Here's how the part is built. I have some questions about the finished solid (model axes, mm). Face numbers are marked on the shaded views. Coordinates: 2 decimals unless noted, no trailing zeros. Write each question's results on one line, items separated by ' | '. Start each with the question number.
from build123d import *

# Parameters (mm, degrees)
F2_R      = 8
F3_DEPTH  = 1
F9_R      = 1
F9_R_2    = 2.6
F10_DEPTH = 5.001


with BuildPart() as f3:
    # F2 (on offset) → F3 (new body)
    with BuildSketch(Plane.XY.offset(-5)):
        Circle(F2_R)
    extrude(amount=F3_DEPTH)

    # F4 (on face) → F5 section 0
    with BuildSketch(Plane.XY.offset(-4)):
        with BuildLine():
            Line((0, 0), (5.6568542495, 5.6568542495))
            ThreePointArc((5.6568542495, 5.6568542495), (3.8674315589, 7.0030688371), (1.775, 7.8006009384))
            ThreePointArc((1.775, 7.8006009384), (0, 8), (-1.775, 7.8006009384))
            ThreePointArc((-1.775, 7.8006009384), (-3.8674315589, 7.0030688371), (-5.6568542495, 5.6568542495))
            Line((-5.6568542495, 5.6568542495), (0, 0))
        make_face()
    # F0 (on Top) → F5 section 1
    with BuildSketch(Plane.XY):
        with BuildLine():
            Line((1.775, 1.775), (1.775, 5.9926517503))
            ThreePointArc((1.775, 5.9926517503), (0, 6.25), (-1.775, 5.9926517503))
            Line((-1.775, 5.9926517503), (-1.775, 1.775))
            Line((-1.775, 1.775), (0, 0))
            Line((0, 0), (1.775, 1.775))
        make_face()
    loft()

    # F4 (on face) → F6 section 0
    with BuildSketch(Plane.XY.offset(-4)):
        with BuildLine():
            Line((-5.6568542495, -5.6568542495), (0, 0))
            Line((0, 0), (-5.6568542495, 5.6568542495))
            ThreePointArc((-5.6568542495, 5.6568542495), (-7.0030688371, 3.8674315589), (-7.8006009384, 1.775))
            ThreePointArc((-7.8006009384, 1.775), (-8, 0), (-7.8006009384, -1.775))
            ThreePointArc((-7.8006009384, -1.775), (-7.0030688371, -3.8674315589), (-5.6568542495, -5.6568542495))
        make_face()
    # F0 (on Top) → F6 section 1
    with BuildSketch(Plane.XY):
        with BuildLine():
            Line((-1.775, -1.775), (0, 0))
            Line((0, 0), (-1.775, 1.775))
            Line((-1.775, 1.775), (-5.9926517503, 1.775))
            ThreePointArc((-5.9926517503, 1.775), (-6.25, 0), (-5.9926517503, -1.775))
            Line((-5.9926517503, -1.775), (-1.775, -1.775))
        make_face()
    loft()

    # F4 (on face) → F7 section 0
    with BuildSketch(Plane.XY.offset(-4)):
        with BuildLine():
            Line((5.6568542495, -5.6568542495), (0, 0))
            Line((0, 0), (-5.6568542495, -5.6568542495))
            ThreePointArc((-5.6568542495, -5.6568542495), (-3.8674315589, -7.0030688371), (-1.775, -7.8006009384))
            ThreePointArc((-1.775, -7.8006009384), (0, -8), (1.775, -7.8006009384))
            ThreePointArc((1.775, -7.8006009384), (3.8674315589, -7.0030688371), (5.6568542495, -5.6568542495))
        make_face()
    # F0 (on Top) → F7 section 1
    with BuildSketch(Plane.XY):
        with BuildLine():
            Line((1.775, -1.775), (0, 0))
            Line((0, 0), (-1.775, -1.775))
            Line((-1.775, -1.775), (-1.775, -5.9926517503))
            ThreePointArc((-1.775, -5.9926517503), (0, -6.25), (1.775, -5.9926517503))
            Line((1.775, -5.9926517503), (1.775, -1.775))
        make_face()
    loft()

    # F4 (on face) → F8 section 0
    with BuildSketch(Plane.XY.offset(-4)):
        with BuildLine():
            ThreePointArc((7.8006009384, 1.775), (7.0030688371, 3.8674315589), (5.6568542495, 5.6568542495))
            Line((5.6568542495, 5.6568542495), (0, 0))
            Line((0, 0), (5.6568542495, -5.6568542495))
            ThreePointArc((5.6568542495, -5.6568542495), (7.0030688371, -3.8674315589), (7.8006009384, -1.775))
            ThreePointArc((7.8006009384, -1.775), (8, 0), (7.8006009384, 1.775))
        make_face()
    # F0 (on Top) → F8 section 1
    with BuildSketch(Plane.XY):
        with BuildLine():
            Line((5.9926517503, 1.775), (1.775, 1.775))
            Line((1.775, 1.775), (0, 0))
            Line((0, 0), (1.775, -1.775))
            Line((1.775, -1.775), (5.9926517503, -1.775))
            ThreePointArc((5.9926517503, -1.775), (6.25, 0), (5.9926517503, 1.775))
        make_face()
    loft()

    # F9 (on Top) → F10 (cut, through all)
    with BuildSketch(Plane.XY):
        with Locations((0, 4.5)):
            Circle(F9_R)
        with Locations((4.5, 0)):
            Circle(F9_R)
        with Locations((0, -4.5)):
            Circle(F9_R)
        with Locations((-4.5, 0)):
            Circle(F9_R)
        Circle(F9_R_2)
    extrude(amount=-F10_DEPTH, mode=Mode.SUBTRACT)


solid = f3.part
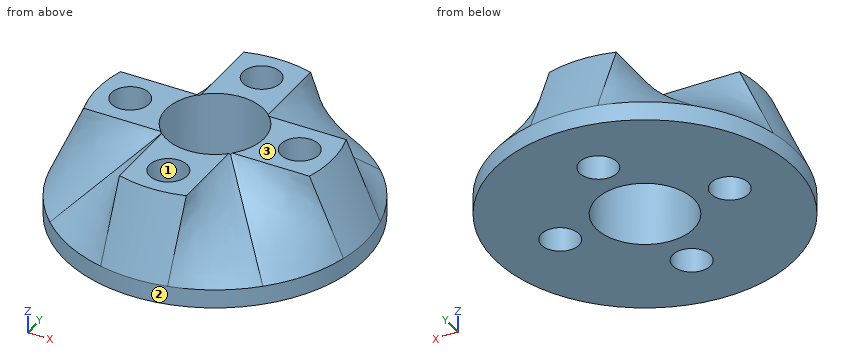
1) I want a section at A-A, the plane x = 0. Give the number of separate pieces and of enclosed holes in the cut face, then the cut area to 3 significant figures.
2) We'd pull the mould along Y, two halves only. Please class the marked faces 1, 2 and 3: pulls with the +Y half, pulls with the -Y half, needs draft (parallel to the pull), parting line crosses it, or undercut.
3) Please list where these lines run through material, in increasing order: line 1 (Y direction, x = 0, z = -1.4); line 2 (Y direction, x = 0, z = -2.4); line 3 (X direction, y = 0.25, z = -3.05). Write a range as [from, to].
4) For pin 1 Ø3 at (x, z) = (-4.5, -4) entering from +Y; pin 2 Ø1 at (x, y) = (2.5, -2.5) entering from +Z; pin 3 Ø4.5 at (x, y) = (0, 0) entering from -Z, each with a flat end and sliding along its axis, tell me the tip position at first contact or that it passes through.
Output:
1) separate pieces: 4 | enclosed holes: 0 | area: 27.0 mm2
2) face 1: undercut | face 2: parting line crosses it | face 3: needs draft
3) line 1: y = [-6.86, -5.5], [-3.5, -2.6], [2.6, 3.5], [5.5, 6.86] | line 2: y = [-7.3, -5.5], [-3.5, -2.6], [2.6, 3.5], [5.5, 7.3] | line 3: x = [-7.58, -5.47], [-3.53, -2.59], [2.59, 3.53], [5.47, 7.58]
4) pin 1: stops at y = 7.42 | pin 2: stops at z = -0.26 | pin 3: passes through
